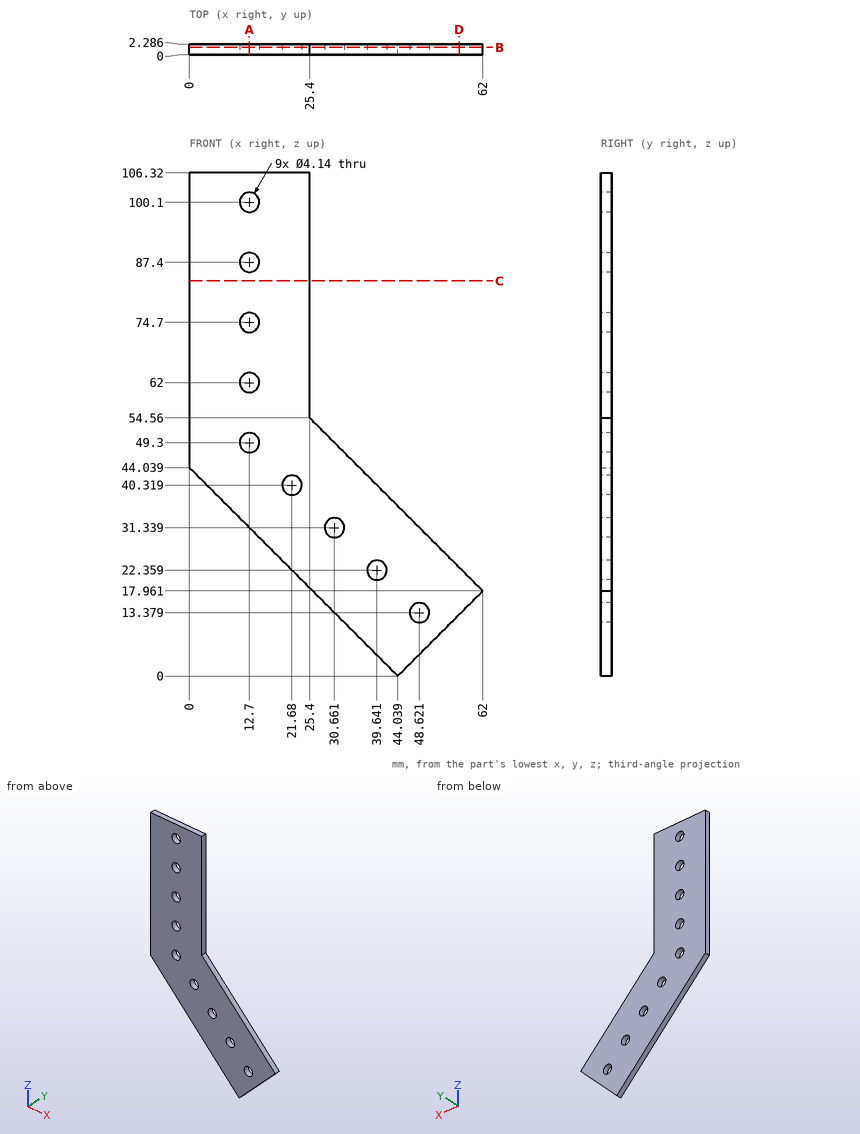
Print and shaded views of the part. All mm, measured from the part's lowest x, y and z. Coordinates: 2 decimals unless noted, no trailing zeros. Loops run counter-clockwise (first coordinate to the right, second up) from the corner with the lowest first, then second, coordinate; pieces in that order, holes last. Notation, with made-up numbers: (6, -33) - (22, -33) arc R20 ccw to (22, -25) - close; hole circle Ø10 at (59.25, 53.5). An arc over 180 degrees is marked (long way). Write item = value, one per line. Start each with the question number.
Item 1: Saw through at A-A, the plane x = 12.7. List the corners of the cut face in (y, z) (1 decimal).
Item 2: Saw through at C-C, the plane z = 83.5. List the corners of the cut face in (x, y) (1 decimal).
Item 3: Saw through at B-B, the plane y = 1.55. State how many separate pieces and enclosed holes the cut face has, then the cut area to 3 significant figures.
Item 4: Wall check: probe 1 along Z at (x, y) = (12.7, 1.75); probe 2 along X at (y, z) = (2.1, 100); probe 3 along X at (y, z) = (1.35, 59). Give the ranges that are in metal, low to high. Write a range as [from, to].
Item 5: Saw through at D-D, the plane x = 57. List the corners of the cut face in (y, z) (1 decimal).
Answers:
q1.outline = (0, 31.3) - (2.3, 31.3) - (2.3, 47.2) - (0, 47.2) - close; (0, 51.4) - (2.3, 51.4) - (2.3, 59.9) - (0, 59.9) - close; (0, 64.1) - (2.3, 64.1) - (2.3, 72.6) - (0, 72.6) - close; (0, 76.8) - (2.3, 76.8) - (2.3, 85.3) - (0, 85.3) - close; (0, 89.5) - (2.3, 89.5) - (2.3, 98) - (0, 98) - close; (0, 102.2) - (2.3, 102.2) - (2.3, 106.3) - (0, 106.3) - close
q2.outline = (0, 0) - (25.4, 0) - (25.4, 2.3) - (0, 2.3) - close
q3.separate_pieces = 1
q3.enclosed_holes = 9
q3.area = 2,780 mm2
q4.probe_1 = [31.34, 47.23], [51.37, 59.93], [64.07, 72.63], [76.77, 85.33], [89.47, 98.03], [102.17, 106.32]
q4.probe_2 = [0, 10.63], [14.77, 25.4]
q4.probe_3 = [0, 25.4]
q5.outline = (0, 13) - (2.3, 13) - (2.3, 23) - (0, 23) - close
